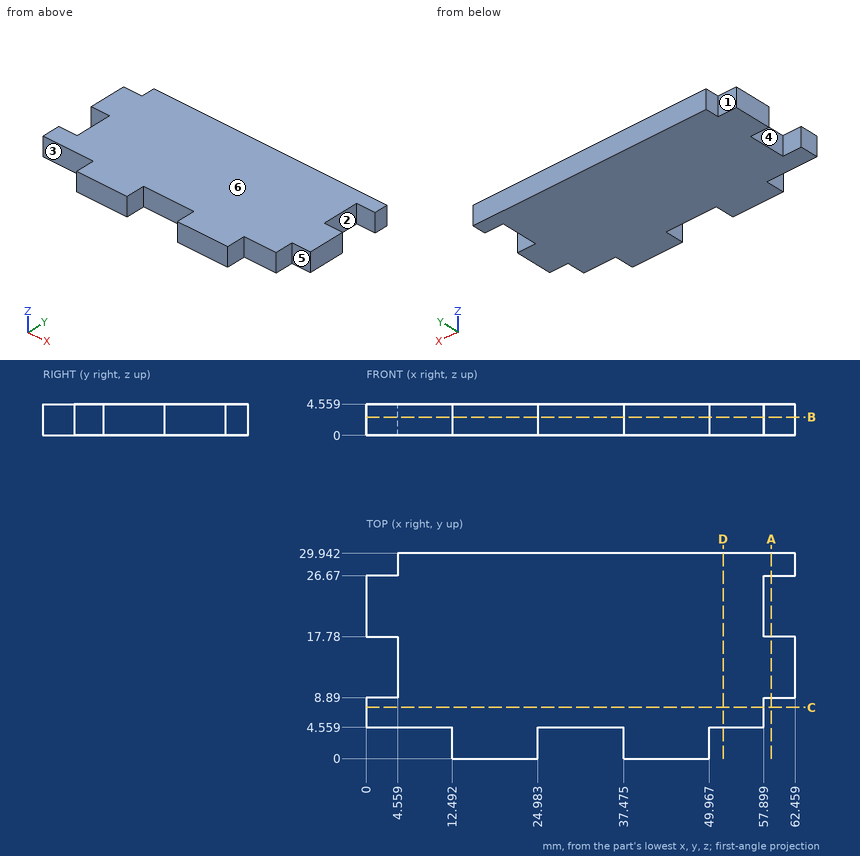
The figure shows three views and two pictorial views of one solid part (mm, origin at its lowest corner). Answer the questions. A direction names the side the tool comes from. Give positions to 0.01 mm unless a question says otherwise; leave off trailing zeros. Write each loop counter-clockwise with the first axis right and the second up, starting at its lowest first coordinate (ties: lowest second). Pieces come first, ordered by that corner, then holes.
Q1. A tool of negligible diameter and unlimited length cuts with its end or side. For the marked faces 1, 2 and 3, from which of +Z, -Z, +X, -X, +Y, -Y can it reach the whole face along a straight path? Write none if from no direction.
Answer:
face 1: +Z, -Z, -X, +Y
face 2: +Z, -Z, +X
face 3: +Z, -Z, -X, -Y
Q2. The part is cut by section D-D on x = 52. Give the vertices of the cut face in (y, z), and give its area (3 significant figures).
Answer:
outline: (4.56, 0) - (29.94, 0) - (29.94, 4.56) - (4.56, 4.56) - close
area: 116 mm2
Q3. The part is cut by section B-B on z = 2.65. Give the vertices of the cut face in (x, y) (1 decimal), and give its area (3 significant figures).
Answer:
outline: (0, 4.6) - (12.5, 4.6) - (12.5, 0) - (25, 0) - (25, 4.6) - (37.5, 4.6) - (37.5, 0) - (50, 0) - (50, 4.6) - (57.9, 4.6) - (57.9, 8.9) - (62.5, 8.9) - (62.5, 17.8) - (57.9, 17.8) - (57.9, 26.7) - (62.5, 26.7) - (62.5, 29.9) - (4.6, 29.9) - (4.6, 26.7) - (0, 26.7) - (0, 17.8) - (4.6, 17.8) - (4.6, 8.9) - (0, 8.9) - close
area: 1,580 mm2
Q4. Given pin 1 (1.4 mm diameter, centred on x = 2.5, z = 3, fed in from -Y); pin 2 (2.5 mm diameter, centred on y = 2.5, z = 1.5, fed in from +X), each flat-ended and moving along its own axis, determine where each tip first touches the part or whether it passes through.
Answer:
pin 1: stops at y = 4.56
pin 2: stops at x = 49.97
Q5. The part is cut by section A-A on x = 59. Give the vertices of the cut face in (y, z).
Answer:
outline: (8.89, 0) - (17.78, 0) - (17.78, 4.56) - (8.89, 4.56) - close; (26.67, 0) - (29.94, 0) - (29.94, 4.56) - (26.67, 4.56) - close
Q6. For a pull along Y with two mould halves and no side action, classify the marked faces 4, 5 and 6 as released by +Y, released by -Y, zero draft, split by the parting line, or undercut.
Answer:
face 4: undercut
face 5: released by -Y
face 6: zero draft
Q7. The part is cut by section C-C on y = 7.5. Give the vertices of the cut face in (x, z), and give its area (3 significant figures).
Answer:
outline: (0, 0) - (57.9, 0) - (57.9, 4.56) - (0, 4.56) - close
area: 264 mm2
Q8. Straight lines are drawn through the part: L1, parallel to Y at x = 4, z = 0.2; L2, parallel to X at y = 19.25, z = 2.1; L3, parallel to X at y = 2.5, z = 0.9 (1 decimal). For each, find the intervals that lie inside material, in ascending order.
Answer:
L1: y = 4.56 to 8.89, 17.78 to 26.67
L2: x = 0 to 57.9
L3: x = 12.5 to 25, 37.5 to 50
